Could you check a few things on this drawing? It's one solid part, dimensions in mm from its lowest x, y, z. A direction names the side the tool comes from. Give positions to 0.01 mm unless a question says otherwise; leave off trailing zeros. Order: outer loops, then holes, each group sorted by start corner. A loop starts at its lowest first (then second) coordinate and runs counter-clockwise, first axis right, second up. Notation, with made-up numbers: M 45.5,46 L 93.5,46 A11 cw 93.5,50 Z; hole C 89.25,71.25 d10. An arc over 180 degrees is marked long. Use one line per item in the form item = value. Start each with the question number.
1. I want a section at B-B, the plane y = 10.25. List the corners of the cut face in (x, z) for me.
2. For the marked faces 4, 5 and 6, which set-ups out of +Z, -Z, +X, -X, +Y, -Y let a thin tool reach every point of the face, with its end or its side?
3. I want a section at C-C, the plane x = 13.5. List the corners of the cut face in (y, z) for me.
4. Will these pins go through, and if not, where does the flat tip stop? P1, Ø12, axis at x = 9.5, y = 10, coming from the -Z side; P2, Ø1, axis at y = 6.5, z = 24, coming from the -X side; P3, Ø3, axis at x = 13, y = 15, coming from the -Z side.
5. We'd pull the mould along Z, two halves only. Please class the marked faces 1, 2 and 3: +Z half, -Z half, draft (parallel to the pull), parting line (faces both ways), or undercut.
6. I need wall thicknesses on L1, parallel to Z at x = 26, y = 17.5; L2, parallel to Z at x = 13, y = 2.25 (1 decimal); L3, parallel to Z at x = 35, y = 4.75. Which ranges of each line are inside material? Lowest first, please.
7. I want a section at A-A, the plane x = 20. List the corners of the cut face in (y, z) for me, and give its area (3 significant figures).
8. I want a section at D-D, the plane x = 30.5. List the corners of the cut face in (y, z) for me, and give its area (3 significant figures).
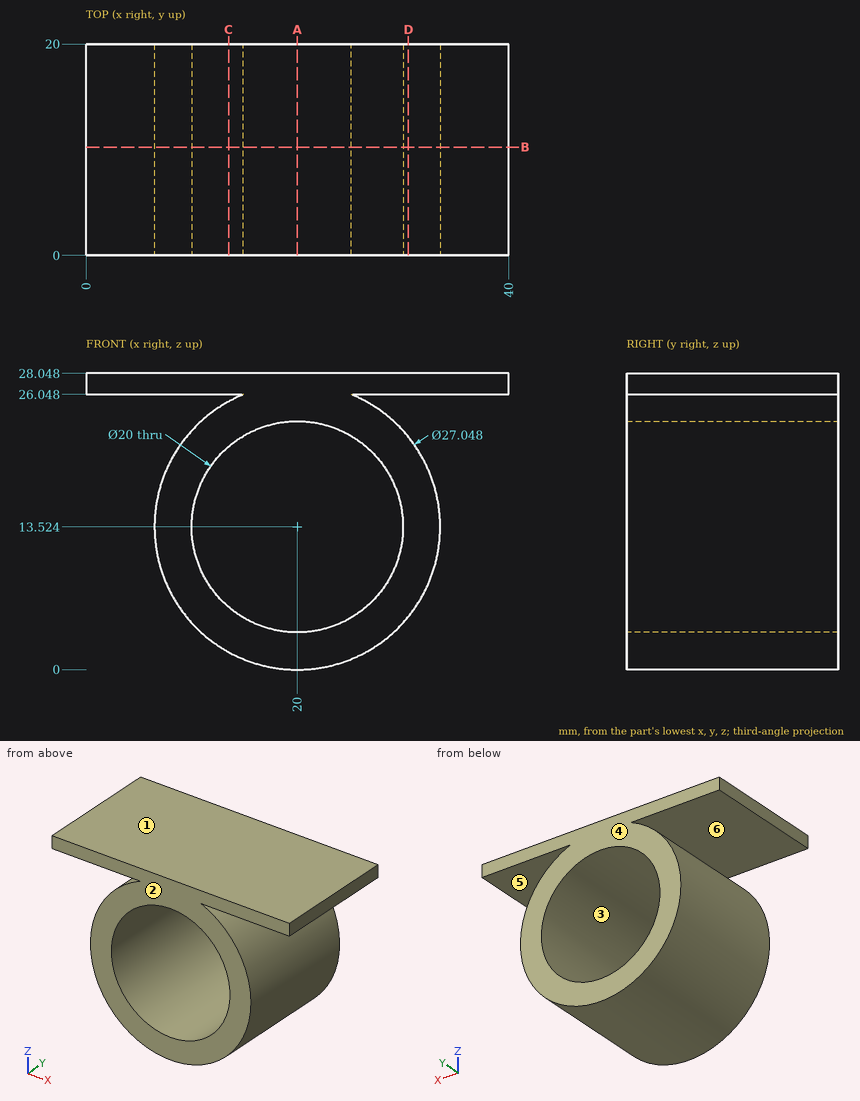
Check result:
q1.outline = M 0,26.05 L 14.9,26.05 A13.52 ccw long 25.1,26.05 L 40,26.05 L 40,28.05 L 0,28.05 Z; hole C 20,13.52 d20
q2.face_4 = +Z, -Z, +X, -X, +Y
q2.face_5 = +X, +Y, -Y
q2.face_6 = -X, +Y, -Y
q3.outline = M 0,1.66 L 20,1.66 L 20,5.92 L 0,5.92 Z; M 0,21.12 L 20,21.12 L 20,25.38 L 0,25.38 Z; M 0,26.05 L 20,26.05 L 20,28.05 L 0,28.05 Z
q4.P1 = 0.77
q4.P2 = 10.87
q4.P3 = 1.17
q5.face_1 = +Z half
q5.face_2 = draft
q5.face_3 = undercut
q6.L1 = 1.4 to 5.52, 21.52 to 25.64, 26.05 to 28.05
q6.L2 = 2 to 6.4, 20.7 to 25.1, 26 to 28
q6.L3 = 26.05 to 28.05
q7.outline = M 0,0 L 20,0 L 20,3.52 L 0,3.52 Z; M 0,23.52 L 20,23.52 L 20,28.05 L 0,28.05 Z
q7.area = 161 mm2
q8.outline = M 0,5 L 20,5 L 20,22.05 L 0,22.05 Z; M 0,26.05 L 20,26.05 L 20,28.05 L 0,28.05 Z
q8.area = 381 mm2
